Part model, mm, in its own coordinate system. A direction names the side the tool comes from. Round coordinates to 2 decimals unless told otherwise and drop trailing zeros. Write each loop counter-clockwise with the first axis right and the second up, starting at its lowest first coordinate (ties: lowest second). Pieces come first, ordered by that corner, then holes. Notation, with made-up numbers: M 66,55 L 75,55 A18 ccw 75,83 Z; hole C 41,-27 d3. An arc over 180 degrees is marked long. Use a Markdown table: item, result. Add a question column.
1) Drop flat-ended pins along their axis: P1, Ø6, axis at x = -2, y = 3.5, coming from the -Z side; P2, Ø2, axis at y = 1, z = -3, coming from the +X side; P3, Ø3, axis at x = -4.5, y = -5, coming from the +Z side. Give the stop position or say it passes through.
2) Wall check: probe 1 along X at (y, z) = (-6.5, 14.5); probe 2 along Z at (x, y) = (9.25, -1.75); probe 3 along Z at (x, y) = (10, 6.25). Give the ranges that are in metal, low to high.
3) Which spindle directions (+Z, -Z, +X, -X, +Y, -Y) get a long thin tool onto all of the face, cutting with end or side? Do faces 4 (the face through (10.7, 0, 17.2)), 5 (the face through (-8, -8.712, 15)), 6 (the face through (1, 0, 5)). Say none if no direction does.
4) Slice it at A-A on y = -6.5. Write the cut outline in (x, z), plus the area to 3 significant figures.
5) Slice it at D-D on x = -4.5. Write the cut outline in (y, z).
6) Two-plate mould, pull along X, no slides. Class faces 1 (the face through (-9.17, 4, 5)), 2 (the face through (7.1, -4.3, 16.9)), 3 (the face through (10.7, 0, -7.7)): released by +X, released by -X, zero draft, split by the parting line, or undercut.
7) Slice it at C-C on z = -6.25. Write the cut outline in (x, y).
8) Slice it at B-B on y = 6.25. Write the cut outline in (x, z).
```python
from build123d import *

# Parameters (mm, degrees)
SKETCH1_W               = 20.3
SKETCH1_H               = 25.7
BOSS_EXTRUDE1_DEPTH     = 7.6708
SKETCH2_R               = 2.5
SKETCH2_R_2             = 1.25
BOSS_EXTRUDE2_DEPTH     = 8.7122
CUT_EXTRUDE1_DEPTH      = 27.682326303
CUT_EXTRUDE1_DEPTH_BACK = 27.682326303
SKETCH3_R               = 1.25


with BuildPart() as part:
    # Sketch1 → Boss-Extrude1 (new body)
    with BuildSketch(Plane(origin=(0, 0, 0), x_dir=(1, 0, 0), z_dir=(0, 1, 0))):
        with Locations((0.979781162, -4.787001603)):
            Rectangle(SKETCH1_W, SKETCH1_H)
    extrude(amount=BOSS_EXTRUDE1_DEPTH)

    # Sketch2 → Boss-Extrude2 (add)
    # profile 1 of 4: a face of its own
    with BuildSketch(Plane(origin=(0, 0, 0), x_dir=(-1, 0, 0), z_dir=(0, -1, 0))):
        with Locations(Location((6.543467427, -15.1920941, 0), (0, 0, 282.050765662))):
            Circle(SKETCH2_R)
        with Locations(Location((6.543467427, -15.1920941, 0), (0, 0, 90))):
            Circle(SKETCH2_R_2, mode=Mode.SUBTRACT)
    # profile 2 of 4: a face of its own
    with BuildSketch(Plane(origin=(0, 0, 0), x_dir=(-1, 0, 0), z_dir=(0, -1, 0))):
        with Locations(Location((-8.925132573, -15.1920941, 0), (0, 0, 257.949234338))):
            Circle(SKETCH2_R)
        with Locations(Location((-8.925132573, -15.1920941, 0), (0, 0, 90))):
            Circle(SKETCH2_R_2, mode=Mode.SUBTRACT)
    # profile 3 of 4: a face of its own
    with BuildSketch(Plane(origin=(0, 0, 0), x_dir=(-1, 0, 0), z_dir=(0, -1, 0))):
        with Locations(Location((-8.925132573, 5.6359059, 0), (0, 0, 208.132514033))):
            Circle(SKETCH2_R)
        with Locations(Location((-8.925132573, 5.6359059, 0), (0, 0, 90))):
            Circle(SKETCH2_R_2, mode=Mode.SUBTRACT)
    # profile 4 of 4: a face of its own
    with BuildSketch(Plane(origin=(0, 0, 0), x_dir=(-1, 0, 0), z_dir=(0, -1, 0))):
        with Locations(Location((6.543467427, 5.6359059, 0), (0, 0, 76.12877324))):
            Circle(SKETCH2_R)
        with Locations(Location((6.543467427, 5.6359059, 0), (0, 0, 90))):
            Circle(SKETCH2_R_2, mode=Mode.SUBTRACT)
    extrude(amount=BOSS_EXTRUDE2_DEPTH)

    # Sketch3 → Cut-Extrude1 (cut, two sides: drawn at the far end of the back side and taken through both)
    with BuildSketch(Plane(origin=(0, 7.6708, 0), x_dir=(1, 0, 0), z_dir=(0, 1, 0)).offset(-CUT_EXTRUDE1_DEPTH_BACK)):
        with Locations(Location((8.925132573, 5.6359059, 0), (0, 0, 270))):
            Circle(SKETCH3_R)
        with Locations(Location((-6.543467427, 5.6359059, 0), (0, 0, 270))):
            Circle(SKETCH3_R)
        with Locations(Location((8.925132573, -15.1920941, 0), (0, 0, 270))):
            Circle(SKETCH3_R)
        with Locations(Location((-6.543467427, -15.1920941, 0), (0, 0, 270))):
            Circle(SKETCH3_R)
    extrude(amount=CUT_EXTRUDE1_DEPTH + CUT_EXTRUDE1_DEPTH_BACK, mode=Mode.SUBTRACT)


solid = part.part
```
Entries:
| question | item | result |
|---|---|---|
| 1 | P1 | stops at z = -8.06 |
| 1 | P2 | stops at x = 11.13 |
| 1 | P3 | stops at z = 17.63 |
| 2 | probe 1 | x = -8.95 to -7.58, -5.5 to -4.14, 6.52 to 7.88, 9.97 to 11.33 |
| 2 | probe 2 | z = -8.11 to -6.84, -4.43 to -3.16, 12.71 to 13.99, 16.4 to 17.67 |
| 2 | probe 3 | z = -8.06 to -6.27, -5 to 14.55, 15.83 to 17.64 |
| 3 | face 4 | +Z, +X, -Y |
| 3 | face 5 | +Z, -Z, +X, -X, -Y |
| 3 | face 6 | -Y |
| 4 | outline | C -6.54,-5.64 d5; C -6.54,15.19 d5; C 8.93,-5.64 d5; C 8.93,15.19 d5; hole C -6.54,-5.64 d2.5; hole C -6.54,15.19 d2.5; hole C 8.93,-5.64 d2.5; hole C 8.93,15.19 d2.5 |
| 4 | area | 58.9 mm^2 |
| 5 | outline | M -8.71,-7.08 L 0,-7.08 L 0,-8.06 L 7.67,-8.06 L 7.67,17.64 L 0,17.64 L 0,16.63 L -8.71,16.63 L -8.71,13.75 L 0,13.75 L 0,-4.2 L -8.71,-4.2 Z |
| 6 | face 1 | released by -X |
| 6 | face 2 | undercut |
| 6 | face 3 | zero draft |
| 7 | outline | M -9.17,0 L -8.97,0 L -8.97,-8.71 L -7.63,-8.71 L -7.63,7.67 L -9.17,7.67 Z; M -5.45,-8.71 L -4.12,-8.71 L -4.12,0 L 6.5,0 L 6.5,-8.71 L 7.84,-8.71 L 7.84,7.67 L -5.45,7.67 Z; M 10.01,-8.71 L 11.35,-8.71 L 11.35,0 L 11.13,0 L 11.13,7.67 L 10.01,7.67 Z |
| 8 | outline | M -9.17,-8.06 L 11.13,-8.06 L 11.13,17.64 L -9.17,17.64 Z; hole C -6.54,-5.64 d2.5; hole C -6.54,15.19 d2.5; hole C 8.93,-5.64 d2.5; hole C 8.93,15.19 d2.5 |
